Geometry: final body of the model. Coordinates: model frame, mm. A direction names the side the tool comes from. Give positions to 0.01 mm unless a question says otherwise; leave off trailing zeros. Write each loop counter-clockwise with the first axis right and the second up, starting at its lowest first coordinate (ties: lowest second). Pieces come first, ordered by that corner, then holes.
Autodesk Inventor part; units mm, degrees
ref_plane "Work Plane1" through (6.2586, 0, 0) normal (0, 0, -1) x (-1, 0, 0)
ref_plane "YZ Plane" through (0, 0, 0) normal (1, 0, 0) x (0, 1, 0)
ref_plane "XZ Plane" through (0, 0, 0) normal (0, 1, 0) x (-1, 0, 0)
sketch "Sketch1" plane through (0, 0, 0) normal (0, 0, 1) x (1, 0, 0)
  line L0 (0, 0) -> (-5, 0)
  line L1 (0, 0) -> (0, 4)
  line L2 (0, 4) -> (-2, 4)
  line L3 (-2, 4) -> (-2, 2.25)
  line L4 (-4, 2.25) -> (-5, 2.25)
  line L5 (-5, 2.25) -> (-5, 0)
  arc A0 (-4, 2.25) -> (-2, 2.25) centre (-3, 3.5036) ccw
  dimension "d0" = 2
  dimension "d1" = 5
  dimension "d2" = 8
  dimension "d3" = 4.5
  dimension "d13" = 3.8
  dimension "d15" = 1
revolve "Body" add sketch "Sketch1" angle 360 about axis through (0, 0, 0) along (-1, 0, 0)
sketch "Sketch2" plane through (-5, 0, 0) normal (-1, 0, 0) x (0, 0, 1)
  circle A0 centre (0, 0) radius 4
  line L0 (0, 0) -> (0, 4) construction
  line L1 (-0.25, 3.9922) -> (0, 3.7422)
  line L2 (0.25, 3.9922) -> (0, 3.7422)
  arc A1 (0.25, 3.9922) -> (-0.25, 3.9922) centre (0, 0) ccw
  circle A2 centre (0, 0) radius 2.25
  dimension "d4" = 90
  dimension "d5" = 0.25
chamfer "Chamfer1" distance 0.2 angle 45 1 edges at (0, -4, 0) measured on face at (0, 0.998, -0.8842)
chamfer "Chamfer2" distance 0.2 angle 45 1 edges at (-2, -4, 0) measured on face at (-2, 3.3779, 0.3191)
extrude "Notch1" [suppressed]
pattern_circular "Notches1" [suppressed]
hole "Thread" at (-5, 0, 0) direction (1, 0, 0) diameter 1.567 end through all
sketch "Sketch4" plane through (-5, 0, 0) normal (-1, 0, 0) x (0, 0, 1)
  circle A0 centre (0, 0) radius 0.7835
  circle A1 centre (0, 0) radius 2.25
  circle A2 centre (0, 0) radius 1.225
  dimension "d42" = 2.45
extrude "Hole1" cut sketch "Sketch4" against normal blind 1.5 contours A2
chamfer "Chamfer3" distance 0.2165 angle 30 1 edges at (-5, 0, -1.225) measured on face at (-5, 1.8836, 0.2287)
ref_plane "Work Plane1" through (6.2586, 0, 0) normal (0, 0, -1) x (-1, 0, 0)
equation "\"d5\" = 0.5 * T"
equation "\"d23\" = PHH"
equation "\"d24\" = FAWI"
equation "\"d38\" = PHH"
equation "\"d25\" = PHH"
equation "\"d26\" = FAWI"
equation "\"d39\" = PHH"
equation "\"d42\" = Da"
equation "\"d43\" = Ta"
equation "\"d10\" = -0.5 * GD1 + 0.5 * NND"
equation "\"d40\" = -0.5 * GD1 + 0.5 * NND"
equation "\"d0\" = KOH1"
equation "\"d1\" = KOH"
equation "\"d2\" = KOD"
equation "\"d3\" = BDM"
equation "\"d13\" = BDMM"
equation "\"d15\" = SLG"
equation "\"FAWI\" = 45deg"
equation "\"T\" = 0.5"
equation "\"NND\" = 2"
equation "\"KOD\" = 8"
equation "\"KOH\" = 5"
equation "\"KOH1\" = 2"
equation "\"BDM\" = 4.5"
equation "\"PHH\" = 0.2"
equation "\"SLG\" = 1"
equation "\"BDMM\" = 3.8"
equation "\"Da\" = 2.45"
equation "\"Ta\" = 1.5"
equation "\"GUL\" = 0.541266 * PTC"
equation "\"RR\" = 1.25"
equation "\"LOTI\" = 1.5"
equation "\"THREADDIA\" = 2"
equation "\"PTC\" = 0.4"
equation "\"GAL\" = 0.541266 * PTC"
equation "\"TOA\" = 30deg"
properties part number "Nut GB 806 M2" material "Steel, Mild"
Q1. Access query for faces 1 (the flat face through (-3.5, -1, 0)), 2 (the cylindrical face through (-1.726, -0.235, 0.747)). Directions: +Z, -Z, +X, -X, +Y, -Y. A direction counts if a zero-diameter tool reaches every point of the face in a straight line with its end or side. Return the directions, or none.
Filled sheet:
face 1: -X
face 2: +X, -X
Q2. Section C-C on x = -1.5. Output: boundary loops of the cut face in (y, z).
Filled sheet:
outline: circle Ø8 at (0, 0); hole circle Ø1.57 at (0, 0)
Q3. Section D-D on x = -2.45. Output: boundary loops of the cut face in (y, z), plus the area to 3 significant figures.
Filled sheet:
outline: circle Ø3.99 at (0, 0); hole circle Ø1.57 at (0, 0)
area: 10.6 mm2
Q4. Ray query, line 1 along Y through (x, z) = (-4.4, 0) (3 decimals); line 2 along Z through (x, y) = (-0.9, 0); line 3 along X through (y, z) = (-0.5, 1). Return the intervals inside material, ascending.
Filled sheet:
line 1: y = -2.25 to -1.225, 1.225 to 2.25
line 2: z = -4 to -0.78, 0.78 to 4
line 3: x = -3.5 to 0
Q5. Pin query (flat end, axial travel): P1, Ø1.2, axis at y = -0.5, z = 0, coming from the -X side; P2, Ø1, axis at x = -4.5, z = 1, coming from the +Y side; P3, Ø1, axis at x = -2, y = 2.5, coming from the +Z side. Return the tip coordinate at first contact, or that it passes through.
Filled sheet:
P1: stops at x = -3.5
P2: stops at y = 2.19
P3: stops at z = 3.44
